Solid Edge part; units mm, degrees
sketch "Sketch1" plane through (0, 0, 0) normal (0, 0, 1) x (1, 0, 0)
  circle A0 centre (0, 0) radius 5.5626
extrude "Protrusion1" add sketch "Sketch1" along normal blind 5.5626
sketch "Sketch2" plane through (0, 0, 0) normal (0, 0, -1) x (0, 1, 0)
  circle A0 centre (0, 0) radius 3.9751
extrude "Protrusion2" add sketch "Sketch2" along normal blind 31.75
sketch "Sketch3" plane through (0, 0, -31.75) normal (0, 0, -1) x (0, 1, 0)
  circle A0 centre (0, 0) radius 3.175
extrude "Protrusion3" add sketch "Sketch3" along normal blind 11.1252
sketch "Sketch4" plane through (0, 0, 5.5626) normal (0, 0, 1) x (0, 1, 0)
  line L0 (-1.9812, 1.0896) -> (0, 2.3891)
  line L1 (-1.9812, -1.2798) -> (-1.9812, 1.0896)
  line L2 (-1.9812, -1.2798) -> (0, -2.3891)
  line L3 (1.9812, -1.2798) -> (0, -2.3891)
  line L4 (1.9812, -1.2798) -> (1.9812, 1.0896)
  line L5 (1.9812, 1.0896) -> (0, 2.3891)
extrude "Cutout1" cut sketch "Sketch4" against normal blind 2.7813
chamfer "Chamfer1" distance 0.7874 angle 45 1 edges at (0, -3.175, -42.8752)
properties part number "24101950"
Could you check a few things on this model? Use its own coordinates, in mm. A direction names the side the tool comes from. Round coordinates to 2 decimals unless told otherwise and drop trailing zeros. Loops run counter-clockwise (first coordinate to the right, second up) from the corner with the lowest first, then second, coordinate; pieces in that order, holes last. Notation, with made-up numbers: M 0,-5.5 L 9,-5.5 A25 cw 9,17.5 Z; hole C -39.5,62 d11. An arc over 180 degrees is marked long. Write item = value, one per line.
1. Will these pins go through, and if not, where does the flat tip stop? P1, Ø2, axis at x = -1.5, z = -36, coming from the -Y side; P2, Ø1.5, axis at y = 1, z = -32, coming from the -X side; P3, Ø5, axis at x = 3, z = -33.5, coming from the -Y side (3 decimals).
Results below:
P1 = -3.14
P2 = -3.96
P3 = -3.785
2. I want a section at A-A, the plane x = 0. Write out the boundary of the cut face in (y, z) (3 decimals).
Results below:
outline = M -5.563,0 L -3.975,0 L -3.975,-31.75 L -3.175,-31.75 L -3.175,-42.088 L -2.388,-42.875 L 2.388,-42.875 L 3.175,-42.088 L 3.175,-31.75 L 3.975,-31.75 L 3.975,0 L 5.563,0 L 5.563,5.563 L 1.981,5.563 L 1.981,2.781 L -1.981,2.781 L -1.981,5.563 L -5.563,5.563 Z
3. I need wall thicknesses on probe 1 along Z at (x, y) = (2, -3); probe 2 along Z at (x, y) = (5.25, -0.25); probe 3 along Y at (x, z) = (2, 3.5). Which ranges of each line are inside material? Lowest first, please.
Results below:
probe_1 = -31.75 to 5.56
probe_2 = 0 to 5.56
probe_3 = -5.19 to -0.69, 0.69 to 5.19
4. Which directions (+Z, -Z, +X, -X, +Y, -Y) give clear straight access to the entire face, cutting with the end or side of a thin tool? Please do faces 5 (the face through (5.306, -1.671, 2.742)), 6 (the face through (3.1, -0.69, -36.85)), 7 (the face through (0, 1.981, 4)).
Results below:
face_5 = +Z, -Z
face_6 = -Z
face_7 = +Z
5. I want a section at C-C, the plane z = -32.5. Write out the boundary of the cut face in (x, y) (3 decimals), and give its area (3 significant figures).
Results below:
outline = C 0,0 d6.35
area = 31.7 mm²
6. I want a section at B-B, the plane z = -8.5. Write out the boundary of the cut face in (x, y).
Results below:
outline = C 0,0 d7.95
7. Thinking about a two-plate mould opening in X: for faces 1 (the face through (-1.73, -1.004, 4.191)), 2 (the face through (0, -1.981, 4)), 3 (the face through (3, -2, -31.75)), 4 (the face through (3.88, -0.86, -15.65)), which applies, +X half, -X half, draft (parallel to the pull), parting line (faces both ways), or undercut?
Results below:
face_1 = undercut
face_2 = undercut
face_3 = draft
face_4 = parting line
